Work out the finished part from the listing and answer in its coordinate system (mm). A direction names the side the tool comes from. Coordinates: 2 decimals unless noted, no trailing zeros. Order: outer loops, then holes, each group sorted by start corner. A loop starts at its lowest first (then second) coordinate and runs counter-clockwise, first axis right, second up. Notation, with made-up numbers: M 65,66.5 L 108,66.5 A34 ccw 108,102.5 Z; hole C -6.5,17 d5. An arc over 180 degrees is marked long. Use a Markdown table: item, result.
from build123d import *

# Parameters (mm, degrees)
BOSS_EXTRUDE2_DEPTH      = 2.5
BOSS_EXTRUDE2_DEPTH_BACK = 2.5


with BuildPart() as part:
    # Sketch1 → Boss-Extrude2 (new, two sides: drawn at the far end of the back side and taken through both)
    with BuildSketch(Plane(origin=(0, 0, 0), x_dir=(1, 0, 0), z_dir=(0, 1, 0)).offset(-BOSS_EXTRUDE2_DEPTH_BACK)):
        with BuildLine():
            Line((-4, 0), (-4, 4))
            Line((-4, 4), (-10, 4))
            Line((-10, 4), (-10, 3))
            Line((-10, 3), (-5, 3))
            Line((-5, 3), (-5, 0))
            ThreePointArc((-5, 0), (0, -5), (5, 0))
            Line((5, 0), (5, 3))
            Line((5, 3), (10, 3))
            Line((10, 3), (10, 4))
            Line((10, 4), (4, 4))
            Line((4, 4), (4, 0))
            ThreePointArc((4, 0), (0, -4), (-4, 0))
        make_face()
    extrude(amount=BOSS_EXTRUDE2_DEPTH + BOSS_EXTRUDE2_DEPTH_BACK)


solid = part.part
1. Section D-D on z = 3.25 is taken. Determine the outline of the cut face in (x, y), then the cut area to 3 significant figures.
Answers below:
| item | result |
|---|---|
| outline | M -3.8,-2.5 L -2.33,-2.5 L -2.33,2.5 L -3.8,2.5 Z; M 2.33,-2.5 L 3.8,-2.5 L 3.8,2.5 L 2.33,2.5 Z |
| area | 14.7 mm² |
2. Find the intervals of material crossed by probe 1 along X at (y, z) = (-1.4, -0.25); probe 2 along X at (y, z) = (-1.85, 3.5); probe 3 along Z at (x, y) = (7, 0.45), in increasing order.
Answers below:
| item | result |
|---|---|
| probe 1 | -5 to -4, 4 to 5 |
| probe 2 | -3.57 to -1.94, 1.94 to 3.57 |
| probe 3 | -4 to -3 |
3. Section B-B on y = 2 is taken. Determine the outline of the cut face in (x, z).
Answers below:
| item | result |
|---|---|
| outline | M -10,-4 L -4,-4 L -4,0 A4 cw 4,0 L 4,-4 L 10,-4 L 10,-3 L 5,-3 L 5,0 A5 ccw -5,0 L -5,-3 L -10,-3 Z |
4. Section A-A on z = 0.5 is taken. Determine the outline of the cut face in (x, y).
Answers below:
| item | result |
|---|---|
| outline | M -4.97,-2.5 L -3.97,-2.5 L -3.97,2.5 L -4.97,2.5 Z; M 3.97,-2.5 L 4.97,-2.5 L 4.97,2.5 L 3.97,2.5 Z |
5. Flat-ended cylindrical pins translate along their axes: P1, Ø2, axis at y = 1, z = -1.5, coming from the -X side; P2, Ø2, axis at x = -4, y = -1, coming from the +Z side; P3, Ø3, axis at y = 0, z = 2.5, coming from the -X side; P4, Ø4, axis at x = -0.5, z = -1.5, coming from the +Y side. Find the tip coordinate at first contact, or state that the pin passes through.
Answers below:
| item | result |
|---|---|
| P1 | x = -5 |
| P2 | z = 4 |
| P3 | x = -4.9 |
| P4 | through |
6. Section C-C on x = 0 is taken. Determine the outline of the cut face in (y, z), then the cut area to 3 significant figures.
Answers below:
| item | result |
|---|---|
| outline | M -2.5,4 L 2.5,4 L 2.5,5 L -2.5,5 Z |
| area | 5.00 mm² |
7. For a pull along X with two mould halves and no side action, classify faces 4 (the face through (0, 0, 5)), 5 (the face through (10, 0, -3.5)), 6 (the face through (0, 0, 4)), 7 (the face through (-4, 2.5, 2)) as +X half, -X half, draft (parallel to the pull), parting line (faces both ways), or undercut.
Answers below:
| item | result |
|---|---|
| face 4 | parting line |
| face 5 | +X half |
| face 6 | undercut |
| face 7 | draft |
8. For faces 1 (the face through (-4, 0, -2)), 2 (the face through (-5, 0, -2)), 3 (the face through (5, 0, -1)), determine the directions among +Z, -Z, +X, -X, +Y, -Y from which every point of the face is accessible in a straight line to the end or side of a thin tool.
Answers below:
| item | result |
|---|---|
| face 1 | -Z, +Y, -Y |
| face 2 | +Z, -X, +Y, -Y |
| face 3 | +Z, +X, +Y, -Y |
